Read the model definition and answer for the solid it produces. Units are mm, in the model's axes. A direction names the side the tool comes from. Round coordinates to 2 decimals unless told otherwise and drop trailing zeros. Order: outer loops, then holes, each group sorted by start corner. A loop starts at its lowest first (then second) coordinate and runs counter-clockwise, first axis right, second up.
from build123d import *

# Parameters (mm, degrees)
SKETCH1_R               = 3.5
SKETCH1_R_2             = 1.498001977
BOSS_EXTRUDE1_DEPTH     = 20.7
SKETCH2_R               = 17.607245412
CUT_EXTRUDE1_DEPTH      = 10.349992
CUT_EXTRUDE2_DEPTH      = 81
CUT_EXTRUDE2_DEPTH_BACK = 81
SKETCH4_R               = 1.498001977
BOSS_EXTRUDE2_DEPTH     = 25.4
CUT_EXTRUDE3_DEPTH      = 8.89
CUT_EXTRUDE4_DEPTH      = 46.1
SKETCH7_R               = 2.286
CUT_EXTRUDE5_DEPTH      = 35.749992


with BuildPart() as part:
    # Sketch1 → Boss-Extrude1 (new body)
    with BuildSketch(Plane(origin=(0, 0, 0), x_dir=(1, 0, 0), z_dir=(0, 1, 0))):
        with BuildLine():
            Line((-58.41, 21.59), (58.41, 21.59))
            ThreePointArc((58.41, 21.59), (80, 0), (58.41, -21.59))
            Line((58.41, -21.59), (-58.41, -21.59))
            ThreePointArc((-58.41, -21.59), (-80, 0), (-58.41, 21.59))
        make_face()
        with Locations((-58.41, 0)):
            Circle(SKETCH1_R, mode=Mode.SUBTRACT)
        with Locations((-51.41, 0)):
            Circle(SKETCH1_R_2, mode=Mode.SUBTRACT)
        with Locations((-65.41, 0)):
            Circle(SKETCH1_R_2, mode=Mode.SUBTRACT)
        with Locations((51.41, 0)):
            Circle(SKETCH1_R_2, mode=Mode.SUBTRACT)
        with Locations((65.41, 0)):
            Circle(SKETCH1_R_2, mode=Mode.SUBTRACT)
        with Locations((58.41, 0)):
            Circle(SKETCH1_R, mode=Mode.SUBTRACT)
    extrude(amount=BOSS_EXTRUDE1_DEPTH)

    # Sketch2 → Cut-Extrude1 (cut)
    with BuildSketch(Plane(origin=(0, 20.7, 0), x_dir=(1, 0, 0), z_dir=(0, 1, 0))):
        with Locations((-58.41, 0)):
            Circle(SKETCH2_R)
    extrude(amount=-CUT_EXTRUDE1_DEPTH, mode=Mode.SUBTRACT)

    # Sketch3 → Cut-Extrude2 (cut, two sides)
    with BuildSketch(Plane(origin=(0, 0, 0), x_dir=(0, 0, -1), z_dir=(1, 0, 0))) as cut_extrude2_sk:
        with BuildLine():
            Line((4.081824225, 10.350008), (-4.081824225, 10.350008))
            ThreePointArc((-4.081824225, 10.350008), (0, 20.065), (4.081824225, 10.350008))
        make_face()
    extrude(amount=CUT_EXTRUDE2_DEPTH, mode=Mode.SUBTRACT)
    extrude(cut_extrude2_sk.sketch, amount=-CUT_EXTRUDE2_DEPTH_BACK, mode=Mode.SUBTRACT)

    # Sketch4 → Boss-Extrude2 (add)
    with BuildSketch(Plane(origin=(0, 20.7, 0), x_dir=(1, 0, 0), z_dir=(0, 1, 0))):
        with BuildLine():
            Line((58.41, -21.59), (58.41, 21.59))
            ThreePointArc((58.41, 21.59), (80, 0), (58.41, -21.59))
        make_face()
        with Locations((65.41, 0)):
            Circle(SKETCH4_R, mode=Mode.SUBTRACT)
    extrude(amount=BOSS_EXTRUDE2_DEPTH)

    # Sketch5 → Cut-Extrude3 (cut)
    with BuildSketch(Plane.ZY.offset(-58.41)):
        with BuildLine():
            Line((0.9525, 22.652744662), (-0.9525, 22.652744662))
            Line((-0.9525, 22.652744662), (-0.9525, 23.922744662))
            ThreePointArc((-0.9525, 23.922744662), (0, 42.925), (0.9525, 23.922744662))
            Line((0.9525, 23.922744662), (0.9525, 22.652744662))
        make_face()
    extrude(amount=-CUT_EXTRUDE3_DEPTH, mode=Mode.SUBTRACT)

    # Sketch6 → Cut-Extrude4 (cut)
    with BuildSketch(Plane(origin=(0, 46.1, 0), x_dir=(1, 0, 0), z_dir=(0, 1, 0))):
        with BuildLine():
            Line((58.41, -3.5), (58.41, 3.5))
            ThreePointArc((58.41, 3.5), (54.91, 0), (58.41, -3.5))
        make_face()
        with BuildLine():
            ThreePointArc((58.41, -3.5), (61.91, 0), (58.41, 3.5))
            Line((58.41, 3.5), (58.41, -3.5))
        make_face()
    extrude(amount=-CUT_EXTRUDE4_DEPTH, mode=Mode.SUBTRACT)

    # Sketch7 → Cut-Extrude5 (cut)
    with BuildSketch(Plane(origin=(0, 46.1, 0), x_dir=(1, 0, 0), z_dir=(0, 1, 0))):
        with Locations((65.41, 0)):
            Circle(SKETCH7_R)
    extrude(amount=-CUT_EXTRUDE5_DEPTH, mode=Mode.SUBTRACT)


solid = part.part
Q1. For faces 1 (the face through (-42.145, 15.597, 6.744)), 2 (the face through (67.3, 34, 5)), 3 (the face through (58.41, 33, -14)), determine the directions among +Z, -Z, +X, -X, +Y, -Y from which every point of the face is accessible in a straight line to the end or side of a thin tool.
Outcome:
face 1: +Y
face 2: -X
face 3: +Z, -Z, -X, +Y
Q2. Straight lines are drawn through the part: probe 1 along Z at (x, y) = (-58, 20.5); probe 2 along Z at (x, y) = (-51.41, 7.75); probe 3 along X at (y, z) = (4, 2). For each, find the intervals that lie inside material, in ascending order.
Outcome:
probe 1: z = -21.59 to -17.6, 17.6 to 21.59
probe 2: z = -21.59 to -1.5, 1.5 to 21.59
probe 3: x = -79.91 to -61.28, -55.54 to 55.54, 61.28 to 79.91
Q3. For a pull along Z with two mould halves and no side action, classify faces 4 (the face through (-23, 10.35, 3)), 5 (the face through (80, 23, 0)), 6 (the face through (69, 46.1, 0)) as released by +Z, released by -Z, zero draft, split by the parting line, or undercut.
Outcome:
face 4: undercut
face 5: split by the parting line
face 6: zero draft
Q4. A cutting plane is placed at B-B, the plane x = 51.41. Give the vertices of the cut face in (y, z) (3 decimals).
Outcome:
outline: (0, -21.59) - (20.7, -21.59) - (20.7, -1.498) - (19.865, -1.498) arc R5.715 cw to (10.35, -4.082) - (10.35, -1.498) - (0, -1.498) - close; (0, 1.498) - (10.35, 1.498) - (10.35, 4.082) arc R5.715 cw to (19.865, 1.498) - (20.7, 1.498) - (20.7, 21.59) - (0, 21.59) - close
Q5. A cutting plane is placed at A-A, the plane y = 3.5. Give the vertices of the cut face in (x, z).
Outcome:
outline: (-58.41, -21.59) - (58.41, -21.59) arc R21.59 ccw to (58.41, 21.59) - (-58.41, 21.59) arc R21.59 ccw to start; hole circle Ø3 at (-65.41, 0); hole circle Ø7 at (-58.41, 0); hole circle Ø3 at (-51.41, 0); hole circle Ø3 at (51.41, 0); hole circle Ø7 at (58.41, 0); hole circle Ø3 at (65.41, 0)
Q6. A cutting plane is placed at C-C, the plane y = 14.35. Give the vertices of the cut face in (x, z) (1 decimal), plus the area to 3 significant figures.
Outcome:
outline: (-79.2, -5.7) arc R21.6 ccw to (-58.4, -21.6) - (58.4, -21.6) arc R21.6 ccw to (79.2, -5.7) - (-41.8, -5.7) arc R17.6 cw to (-75.1, -5.7) - close; (-79.2, 5.7) - (-75.1, 5.7) arc R17.6 cw to (-41.8, 5.7) - (79.2, 5.7) arc R21.6 ccw to (58.4, 21.6) - (-58.4, 21.6) arc R21.6 ccw to start
area: 4,110 mm2
Q7. Flat-ended cylindrical pins translate along their axes: pin 1 (3 mm diameter, centred on y = 13, z = 5, fed in from +X); pin 2 (15 mm diameter, centred on y = 33.4, z = 0, fed in from -X); pin 3 (3.5 mm diameter, centred on x = 51.41, z = 0, fed in from +Y). Find the tip coordinate at first contact, or state that the pin passes through.
Outcome:
pin 1: stops at x = 79.42
pin 2: stops at x = 67.3
pin 3: stops at y = 20.7
Q8. A cutting plane is placed at D-D, the plane y = 33.4. Give the vertices of the cut face in (x, z) (3 decimals), plus the area to 3 significant figures.
Outcome:
outline: (58.41, -21.59) arc R21.59 ccw to (58.41, 21.59) - (58.41, 9.525) - (67.3, 9.525) - (67.3, 1.286) arc R2.286 cw to (67.3, -1.286) - (67.3, -9.525) - (58.41, -9.525) - close
area: 562 mm2
